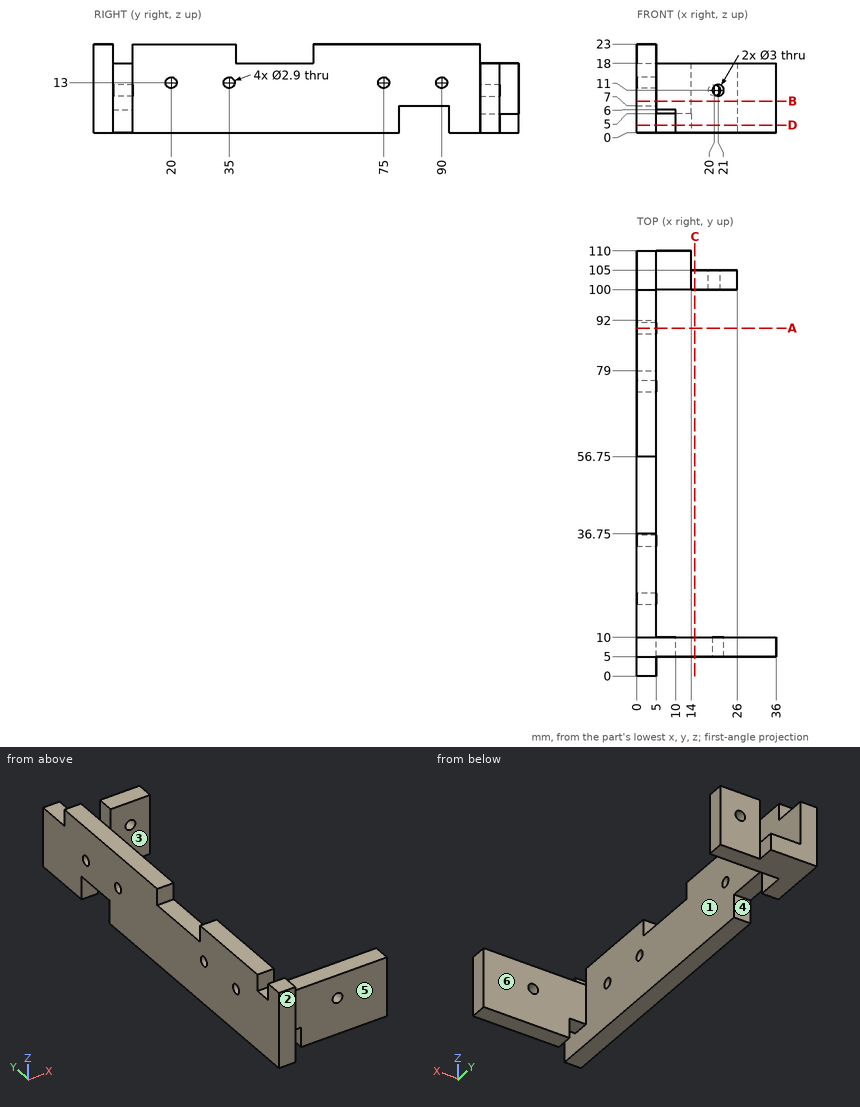
Source: three-view drawing plus pictorial views. Frame: mm from the lowest corner of the part. A direction names the side the tool comes from. Round coordinates to 2 decimals unless told otherwise and drop trailing zeros. Loops run counter-clockwise (first coordinate to the right, second up) from the corner with the lowest first, then second, coordinate; pieces in that order, holes last. Notation, with made-up numbers: (28, 1) -> (60, 1) arc R12 cw to (60, 20) -> close; hole circle Ø8 at (-11.5, 79). An arc over 180 degrees is marked (long way). Use one line per item in the form item = value.
Item 1: Draft query along Y for the marked faces 1, 2 and 3. Return one class per face: released by +Y, released by -Y, zero draft, split by the parting line, or undercut.
Evaluation:
face_1 = zero draft
face_2 = released by -Y
face_3 = undercut
Item 2: Access query for the marked faces 4, 5 and 6. Directions: +Z, -Z, +X, -X, +Y, -Y. A direction counts if a zero-diameter tool reaches every point of the face in a straight line with its end or side. Return the directions, or none.
Evaluation:
face_4 = -Z, +X, -X
face_5 = +Z, -Z, +X, -Y
face_6 = +Z, -Z, +X
Item 3: Contact query for flat-ended pins moving along their axis: pin 1 Ø5.5 at (x, z) = (15.5, 6) entering from -Y; pin 2 Ø5.5 at (x, z) = (2, 21) entering from +Y; pin 3 Ø1.5 at (x, y) = (3.5, 86) entering from -Z; pin 4 Ø1 at (x, y) = (9.5, 11.5) entering from -Z. Output: stop coordinate, or through.
Evaluation:
pin_1 = 5
pin_2 = 100
pin_3 = 7
pin_4 = through
Item 4: Cut plane C-C on x = 15. Output: boundary loops of the cut face in (y, z), then the cut area to 3 significant figures.
Evaluation:
outline = (5, 0) -> (10, 0) -> (10, 18) -> (5, 18) -> close; (100, 0) -> (105, 0) -> (105, 18) -> (100, 18) -> close
area = 180 mm2
Item 5: Cut plane A-A on y = 90. Output: boundary loops of the cut face in (x, z).
Evaluation:
outline = (0, 7) -> (5, 7) -> (5, 11.55) -> (0, 11.55) -> close; (0, 14.45) -> (5, 14.45) -> (5, 23) -> (0, 23) -> close
Item 6: Cut plane B-B on z = 8.25. Output: boundary loops of the cut face in (x, y).
Evaluation:
outline = (0, 0) -> (5, 0) -> (5, 5) -> (36, 5) -> (36, 10) -> (5, 10) -> (5, 110) -> (0, 110) -> close; (14, 100) -> (26, 100) -> (26, 105) -> (14, 105) -> close
Item 7: Material intervals for probe 1 along Y at (x, z) = (15.5, 9); probe 2 along Z at (x, y) = (2.8, 90); probe 3 along Z at (x, y) = (2, 35), sorted ascending.
Evaluation:
probe_1 = 5 to 10, 100 to 105
probe_2 = 7 to 11.55, 14.45 to 23
probe_3 = 0 to 11.55, 14.45 to 23
Item 8: Cut plane D-D on z = 2. Output: boundary loops of the cut face in (x, y), then the cut area to 3 significant figures.
Evaluation:
outline = (0, 0) -> (5, 0) -> (5, 79) -> (0, 79) -> close; (0, 92) -> (5, 92) -> (5, 100) -> (26, 100) -> (26, 105) -> (14, 105) -> (14, 110) -> (0, 110) -> close; (10, 5) -> (36, 5) -> (36, 10) -> (10, 10) -> close
area = 765 mm2
